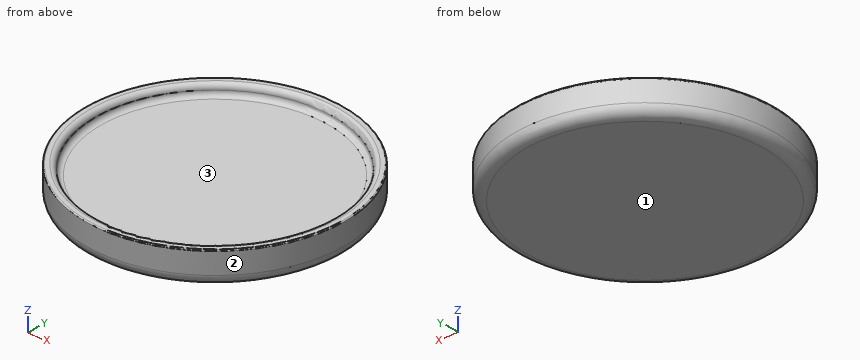
```python
from build123d import *

# Parameters (mm, degrees)
SKETCH1_R          = 127
BASE_EXTRUDE_DEPTH = 31.75
SKETCH3_R          = 117
CUT_EXTRUDE1_DEPTH = 10
FILLET1_R          = 5
FILLET2_R          = 5
FILLET3_R          = 1
FILLET4_R          = 10
SCALE2_SCALE       = 1.2


with BuildPart() as part:
    # Sketch1 → Base-Extrude (new body)
    with BuildSketch(Plane.XY):
        Circle(SKETCH1_R)
    extrude(amount=-BASE_EXTRUDE_DEPTH)

    # Sketch3 → Cut-Extrude1 (cut)
    with BuildSketch(Plane.XY):
        Circle(SKETCH3_R)
    extrude(amount=-CUT_EXTRUDE1_DEPTH, mode=Mode.SUBTRACT)

    # Fillet1
    fillet1_edges = [part.edges().sort_by_distance(p)[0] for p in [
        (-117, 0, 0),
    ]]
    fillet(fillet1_edges, radius=FILLET1_R)

    # Fillet2
    fillet2_edges = [part.edges().sort_by_distance(p)[0] for p in [
        (-117, 0, -10),
    ]]
    fillet(fillet2_edges, radius=FILLET2_R - 0.0001)  # a hair under: the kernel refuses the full size

    # Fillet3
    fillet3_edges = [part.edges().sort_by_distance(p)[0] for p in [
        (-127, 0, 0),
    ]]
    fillet(fillet3_edges, radius=FILLET3_R)

    # Fillet4
    fillet4_edges = [part.edges().sort_by_distance(p)[0] for p in [
        (-127, 0, -31.75),
    ]]
    fillet(fillet4_edges, radius=FILLET4_R)


with BuildPart() as part_1:
    # Scale2: scaled about (0, 0, -19.732997693)
    add(part.part.scale(SCALE2_SCALE).moved(Location((0, 0, 3.946599539))))


solid = part_1.part
```
The model under review builds one solid part; all positions refer to its coordinate system, in mm. Face numbers are marked on the shaded views. Coordinates: 2 decimals unless noted, no trailing zeros. Write each loop counter-clockwise with the first axis right and the second up, starting at its lowest first coordinate (ties: lowest second). Pieces come first, ordered by that corner, then holes. Notation, with made-up numbers: (14.25, 24) - (36.25, 24) arc R11 ccw to (36.25, 35) - close; hole circle Ø6 at (-10.75, 84). An arc over 180 degrees is marked (long way). Answer in a Markdown table with one row per item. Add a question column.
Q1. To check wall thickness, follow line 1 along Y through (x, z) = (0, -2); line 2 along Y through (x, z) = (108.5, -5.5); line 3 along Z through (x, y) = (-74, -105.5). State the ranges of each line that lie inside material, in increasing order. Write a range as from..to.
Q2. Clearance check with flat-ended pins moving along their axes: pin 1 (4 mm diameter, centred on y = -112, z = -10, fed in from +X); pin 2 (5 mm diameter, centred on x = 98, z = -0.5, fed in from +Y); pin 3 (8 mm diameter, centred on x = -97, z = -14, fed in from +Y). State where each tip first meets the part, or that it passes through.
Q3. Consider section C-C on z = -13.5. Give the boundary of the cut face in (x, y).
Q4. Draft analysis for pull direction Y (two halves, no side actions). For the marked faces 1, 2 and 3, state which applies: +Y half, -Y half, draft (parallel to the pull), parting line (faces both ways), or undercut.
Answers below:
| question | item | result |
|---|---|---|
| 1 | line 1 | -152.4..-140.4, 140.4..152.4 |
| 1 | line 2 | -107.02..-87.38, 87.38..107.02 |
| 1 | line 3 | -34.15..-8.05 |
| 2 | pin 1 | x = 105.48 |
| 2 | pin 2 | y = 118.77 |
| 2 | pin 3 | y = 120.73 |
| 3 | outline | circle Ø304.8 at (0, 0) |
| 4 | face 1 | draft |
| 4 | face 2 | parting line |
| 4 | face 3 | undercut |
